Answer from the drawing. Dimensions are ordinates in mm from the lowest x, y and z of the part. A direction names the side the tool comes from. Round coordinates to 2 decimals unless told otherwise and drop trailing zeros. Loops run counter-clockwise (first coordinate to the right, second up) from the corner with the lowest first, then second, coordinate; pieces in that order, holes last.
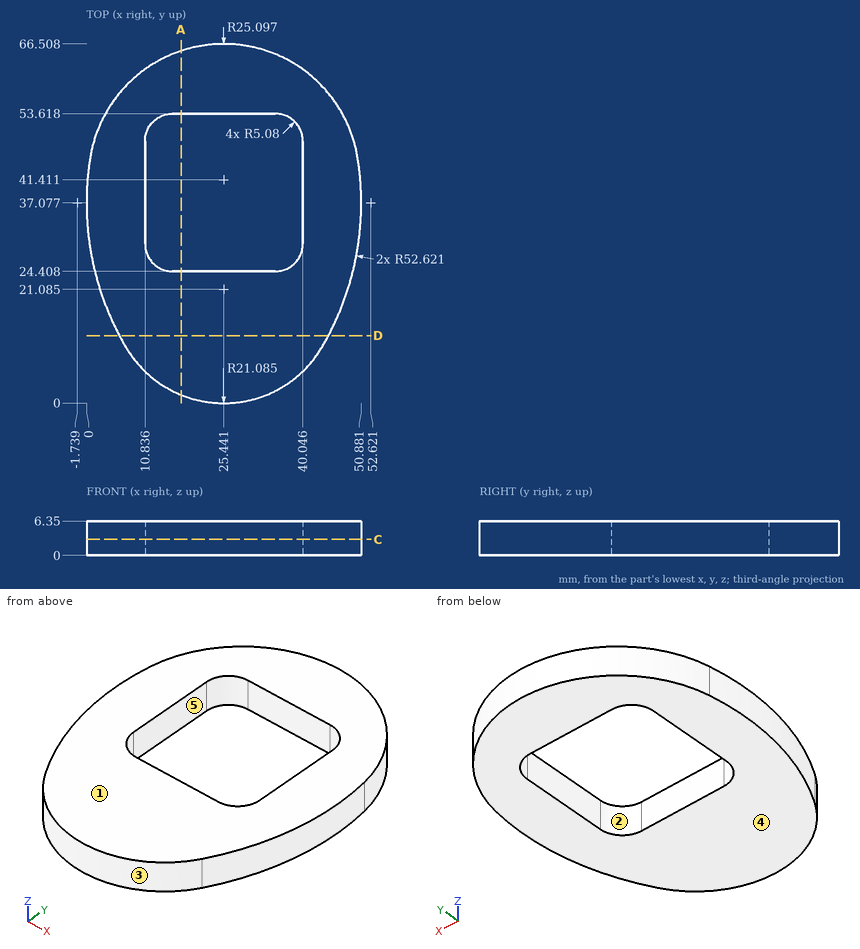
1. Determine the mould class of the marked faces 3, 4 and 5 for opening direction X: +X half, -X half, draft (parallel to the pull), parting line (faces both ways), or undercut.
Answer key:
face 3: parting line
face 4: draft
face 5: undercut
2. Consider probe 1 along X at (y, z) = (37.5, 4.25) (1 decimal); probe 2 along X at (y, z) = (45, 5.75) (1 decimal); probe 3 along Y at (x, z) = (29.5, 4.25) (1 decimal). Determine where each line is inside the solid, lowest interval first.
Answer key:
probe 1: x = 0 to 10.8, 40 to 50.9
probe 2: x = 0.6 to 10.8, 40 to 50.3
probe 3: y = 0.4 to 24.4, 53.6 to 66.2
3. Find section C-C (z = 3). Write down the section's boundary in (x, y) (1 decimal), then the cut area to 3 significant figures.
Answer key:
outline: (0.7, 45.4) arc R52.6 ccw to (7.3, 10.4) arc R21.1 ccw to (43.6, 10.4) arc R52.6 ccw to (50.2, 45.4) arc R25.1 ccw to start; hole (10.8, 29.5) arc R5.1 ccw to (15.9, 24.4) - (35, 24.4) arc R5.1 ccw to (40, 29.5) - (40, 48.5) arc R5.1 ccw to (35, 53.6) - (15.9, 53.6) arc R5.1 ccw to (10.8, 48.5) - close
area: 1,880 mm2
4. Given pin 1 (3 mm diameter, centred on x = 23.5, z = 4.5, fed in from +Y); pin 2 (1 mm diameter, centred on x = 31.5, y = 14, fed in from -Z); pin 3 (1.9 mm diameter, centred on x = 28.5, z = 3.5, fed in from -Y); pin 4 (1.5 mm diameter, centred on y = 39.5, z = 5.5, fed in from +X), each flat-ended and moving along its own axis, determine where each tip first touches the part or whether it passes through.
Answer key:
pin 1: stops at y = 66.5
pin 2: stops at z = 0
pin 3: stops at y = 0.11
pin 4: stops at x = 50.85
5. Which of the six approach directions +Z, -Z, +X, -X, +Y, -Y give full straight-line access (tool end or side, diameter ignored) to the marked faces 1 and 2?
Answer key:
face 1: +Z, +X, -X, +Y, -Y
face 2: +Z, -Z
6. Find section D-D (y = 12.5). Write down the section's boundary in (x, z).
Answer key:
outline: (6.09, 0) - (44.79, 0) - (44.79, 6.35) - (6.09, 6.35) - close
7. Find section A-A (x = 17.5). Write down the section's boundary in (y, z).
Answer key:
outline: (1.55, 0) - (24.41, 0) - (24.41, 6.35) - (1.55, 6.35) - close; (53.62, 0) - (65.22, 0) - (65.22, 6.35) - (53.62, 6.35) - close
